Read the model definition and answer for the solid it produces. Units are mm, in the model's axes. A direction names the side the tool comes from. Coordinates: 2 decimals unless noted, no trailing zeros. Answer as a JSON object with one key per item and string values. Group by question number.
(1) Which of the six approach directions +Z, -Z, +X, -X, +Y, -Y give full straight-line access (tool end or side, diameter ignored) to faces 1 (the face through (-15.55, 7.99, -8.54)), 2 (the face through (19.305, 15.399, 3.414)), 3 (the face through (8, 11, 8.712))?
(2) Straight lines are drawn through the part: L1, parallel to X at y = 7.5, z = 12.75 (3 decimals); L2, parallel to Z at x = 15.5, y = 8.75; L3, parallel to Z at x = 13, y = 10.75. For each, find the intervals that lie inside material, in ascending order.
(3) For a pull along Y with two mould halves and no side action, classify faces 4 (the face through (17.679, 11, 10)), 5 (the face through (19.305, 0.601, 7.722)), 6 (the face through (-14.125, 3, -1)) as +Y half, -Y half, draft (parallel to the pull), parting line (faces both ways), or undercut.
(4) Flat-ended cylindrical pins translate along their axes: P1, Ø1.4, axis at y = 8.5, z = 10, coming from the +X side; P2, Ø1, axis at y = 12.5, z = 10, coming from the -X side; P3, Ø1, axis at x = 8, y = 11.5, coming from the -Z side. Find the tip coordinate at first contact, or state that the pin passes through.
from build123d import *

# Parameters (mm, degrees)
SALIENTE_EXTRUIR1_DEPTH = 16
CROQUIS5_R              = 5.7
CORTAR_EXTRUIR1_DEPTH   = 38
SALIENTE_EXTRUIR2_DEPTH = 0.6
CORTAR_EXTRUIR2_DEPTH   = 10
REDONDEO1_R             = 7
REDONDEO2_R             = 2
REDONDEO3_R             = 1
REDONDEO5_R             = 1
SALIENTE_EXTRUIR3_START = -2
CROQUIS10_R             = 5.7
CROQUIS10_R_2           = 4.7
SALIENTE_EXTRUIR3_DEPTH = 2


with BuildPart() as part:
    # Croquis1 → Saliente-Extruir1 (new body)
    with BuildSketch(Plane(origin=(0, 0, 0), x_dir=(1, 0, 0), z_dir=(0, 1, 0))):
        with BuildLine():
            Line((-16.125, 9.1375), (19.875, 9.1375))
            Line((19.875, 9.1375), (19.875, -18.8625))
            Line((19.875, -18.8625), (3.603278106, -18.8625))
            Line((3.603278106, -18.8625), (3.603278106, -16.9125))
            ThreePointArc((3.603278106, -16.9125), (3.593299591, -16.727049938), (3.563479273, -16.543741332))
            ThreePointArc((3.563479273, -16.543741332), (1.875, -8.8125), (0.186520727, -16.543741332))
            ThreePointArc((0.186520727, -16.543741332), (0.156700409, -16.727049938), (0.146721894, -16.9125))
            Line((0.146721894, -16.9125), (0.146721894, -18.8625))
            Line((0.146721894, -18.8625), (-16.125, -18.8625))
            Line((-16.125, -18.8625), (-16.125, 9.1375))
        make_face()
    extrude(amount=SALIENTE_EXTRUIR1_DEPTH)

    # Croquis5 → Cortar-Extruir1 (cut)
    with BuildSketch(Plane(origin=(19.875, 0, 0), x_dir=(0, 0, -1), z_dir=(1, 0, 0))):
        with Locations((0.6375, 8)):
            Circle(CROQUIS5_R)
    extrude(amount=-CORTAR_EXTRUIR1_DEPTH, mode=Mode.SUBTRACT)

    # Croquis8 → Saliente-Extruir2 (add)
    with BuildSketch(Plane.XZ):
        with BuildLine():
            Line((-2.175, 12.8625), (5.925, 12.8625))
            ThreePointArc((5.925, 12.8625), (1.875, 8.8125), (-2.175, 12.8625))
        make_face()
    extrude(amount=-SALIENTE_EXTRUIR2_DEPTH)

    # Croquis9 → Cortar-Extruir2 (cut)
    with BuildSketch(Plane(origin=(0, 16, 0), x_dir=(1, 0, 0), z_dir=(0, 1, 0))):
        Polygon((-15.929202857, -9.7125), (-15.929202857, -10.9625), (-16.125, -10.9625), (-16.125, -8.8125), (-5.179202857, -8.7125), (-2.700687259, -8.7125), (-6.793467705, -18.842487075), (-9.112924295, -18.842487075), (-5.929202857, -10.9625), (-7.179202857, -10.9625), (-7.179202857, -9.7125), (-7.929202857, -9.7125), (-7.929202857, -10.9625), (-9.179202857, -10.9625), (-9.179202857, -9.7125), (-9.929202857, -9.7125), (-9.929202857, -10.9625), (-11.179202857, -10.9625), (-11.179202857, -9.7125), (-11.929202857, -9.7125), (-11.929202857, -10.9625), (-13.179202857, -10.9625), (-13.179202857, -9.7125), (-13.929202857, -9.7125), (-13.929202857, -10.9625), (-15.179202857, -10.9625), (-15.179202857, -9.7125), align=None)
        Polygon((12.862924295, -18.842487075), (10.543467705, -18.842487075), (6.450687259, -8.7125), (8.929202857, -8.7125), (19.875, -8.8125), (19.875, -10.9625), (19.679202857, -10.9625), (19.679202857, -9.7125), (18.929202857, -9.7125), (18.929202857, -10.9625), (17.679202857, -10.9625), (17.679202857, -9.7125), (16.929202857, -9.7125), (16.929202857, -10.9625), (15.679202857, -10.9625), (15.679202857, -9.7125), (14.929202857, -9.7125), (14.929202857, -10.9625), (13.679202857, -10.9625), (13.679202857, -9.7125), (12.929202857, -9.7125), (12.929202857, -10.9625), (11.679202857, -10.9625), (11.679202857, -9.7125), (10.929202857, -9.7125), (10.929202857, -10.9625), (9.679202857, -10.9625), align=None)
    extrude(amount=-CORTAR_EXTRUIR2_DEPTH, mode=Mode.SUBTRACT)

    # Redondeo1
    redondeo1_edges = [part.edges().sort_by_distance(p)[0] for p in [
        (1.875, 16, -9.1375),
        (1.875, 0, -9.1375),
    ]]
    fillet(redondeo1_edges, radius=REDONDEO1_R)

    # Redondeo2
    redondeo2_edges = [part.edges().sort_by_distance(p)[0] for p in [
        (19.875, 16, 3.3375),
        (-16.125, 16, 3.3375),
        (-16.125, 8, -9.1375),
        (-16.125, 0, 8.3625),
        (-16.125, 2.050252532, -7.087247468),
        (-16.125, 13.949747468, -7.087247468),
        (19.875, 8, -9.1375),
        (19.875, 2.050252532, -7.087247468),
        (19.875, 13.949747468, -7.087247468),
        (19.875, 0, 8.3625),
    ]]
    fillet(redondeo2_edges, radius=REDONDEO2_R)

    # Redondeo3
    redondeo3_edges = [part.edges().sort_by_distance(p)[0] for p in [
        (1.875, 16, 8.8125),
    ]]
    fillet(redondeo3_edges, radius=REDONDEO3_R)

    # Redondeo5
    redondeo5_edges = [part.edges().sort_by_distance(p)[0] for p in [
        (10.739139053, 0, 18.8625),
        (19.289213562, 0.585786438, 18.8625),
        (-6.989139053, 0, 18.8625),
        (-15.539213562, 0.585786438, 18.8625),
        (19.875, 9, 18.8625),
        (-16.125, 9, 18.8625),
        (-16.125, 16, 14.9125),
        (19.875, 16, 14.9125),
    ]]
    fillet(redondeo5_edges, radius=REDONDEO5_R)

    # Croquis10 → Saliente-Extruir3 (add)
    with BuildSketch(Plane.ZY.offset(16.125).offset(SALIENTE_EXTRUIR3_START)):
        with Locations(Location((-0.6375, 8, 0), (0, 0, 180))):
            Circle(CROQUIS10_R)
        with Locations((-0.6375, 8)):
            Circle(CROQUIS10_R_2, mode=Mode.SUBTRACT)
    extrude(amount=SALIENTE_EXTRUIR3_DEPTH)


solid = part.part
Results below:
{
 "1": {"face 1": "-Z, -X, +Y, -Y", "face 2": "-Z, +X, +Y", "face 3": "+Y"},
 "2": {"L1": "x = -16.125 to -6.651, -4.332 to -2.173, 5.923 to 8.082, 10.401 to 19.875", "L2": "z = -9.14 to -6.29, 5.01 to 8.77, 9.71 to 18.86", "L3": "z = -8.92 to -5.63, 4.36 to 8.75, 9.71 to 18.86"},
 "3": {"face 4": "draft", "face 5": "-Y half", "face 6": "undercut"},
 "4": {"P1": "stops at x = 19.68", "P2": "stops at x = -15.93", "P3": "stops at z = -8.85"}
}
